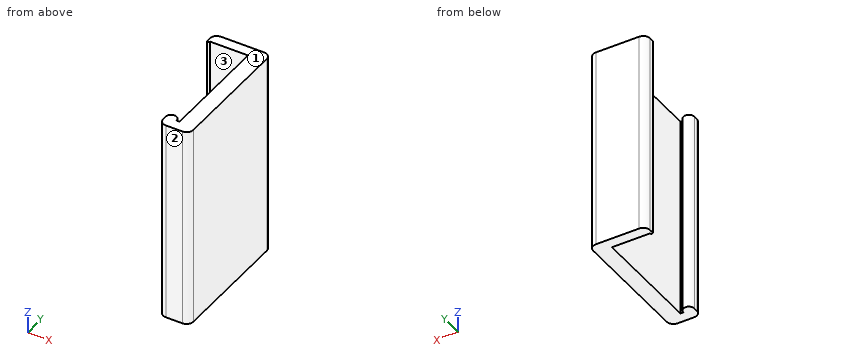
```python
from build123d import *

# Parameters (mm, degrees)
BOSS_EXTRUDE1_DEPTH      = 7.5
BOSS_EXTRUDE1_DEPTH_BACK = 7.5
FILLET1_R                = 0.5


with BuildPart() as part:
    # Sketch2 → Boss-Extrude1 (new, two sides: drawn at the far end of the back side and taken through both)
    with BuildSketch(Plane.XY.offset(-BOSS_EXTRUDE1_DEPTH_BACK)):
        Polygon((37.341321959, 6.45), (40.341321959, 6.45), (40.341321959, -1.8), (39.316321959, -1.8), (39.316321959, -2.6), (41.541321959, -2.6), (41.541321959, 7.25), (37.341321959, 7.25), align=None)
        with BuildLine():
            Line((37.541321959, 6.45), (37.341321959, 6.45))
            ThreePointArc((37.341321959, 6.45), (37.441321959, 6.35), (37.541321959, 6.45))
        make_face()
        with BuildLine():
            ThreePointArc((40.116321959, -1.8), (39.716321959, -1.4), (39.316321959, -1.8))
            Line((39.316321959, -1.8), (40.116321959, -1.8))
        make_face()
    extrude(amount=BOSS_EXTRUDE1_DEPTH + BOSS_EXTRUDE1_DEPTH_BACK)

    # Fillet1
    fillet1_edges = [part.edges().sort_by_distance(p)[0] for p in [
        (37.341321959, 7.25, 0),
        (41.541321959, 7.25, 0),
        (41.541321959, -2.6, 0),
        (39.316321959, -2.6, 0),
    ]]
    fillet(fillet1_edges, radius=FILLET1_R)


solid = part.part
```
Geometry check sheet. Reference: the model listing, model coordinates, mm. Face numbers are marked on the shaded views. Give positions to 0.01 mm unless a question says otherwise; leave off trailing zeros. Write each loop counter-clockwise with the first axis right and the second up, starting at its lowest first coordinate (ties: lowest second). Pieces come first, ordered by that corner, then holes. Notation, with made-up numbers: (2.25, 13) -> (17.25, 13) arc R26 cw to (17.25, 46) -> close; hole circle Ø8 at (37, 88.25). An arc over 180 degrees is marked (long way). Use one line per item in the form item = value.
Item 1: Sectioned sample at A-A on z = 6.5. Enter the section's corners in (x, y), plus the area to 3 significant figures.
Results list:
outline = (37.34, 6.45) arc R0.1 ccw to (37.54, 6.45) -> (40.34, 6.45) -> (40.34, -1.8) -> (40.12, -1.8) arc R0.4 ccw to (39.32, -1.8) -> (39.32, -2.1) arc R0.5 ccw to (39.82, -2.6) -> (41.04, -2.6) arc R0.5 ccw to (41.54, -2.1) -> (41.54, 6.75) arc R0.5 ccw to (41.04, 7.25) -> (37.84, 7.25) arc R0.5 ccw to (37.34, 6.75) -> close
area = 15.1 mm2
Item 2: Sectioned sample at B-B on x = 38.5. Enter the section's corners in (y, z), plus the area to 3 significant figures.
Results list:
outline = (6.45, -7.5) -> (7.25, -7.5) -> (7.25, 7.5) -> (6.45, 7.5) -> close
area = 12.0 mm2
Item 3: Scan lines: line 1 (Y direction, x = 39.75, z = -6.5); line 2 (X direction, y = 3.5, z = -3.5); line 3 (Y direction, x = 37.8, z = -6.25). Record each from-to range of solid material in increasing order.
Results list:
line_1 = -2.6 to -1.4, 6.45 to 7.25
line_2 = 40.34 to 41.54
line_3 = 6.45 to 7.25
Item 4: Sectioned sample at C-C on y = 1.5. Enter the section's corners in (x, z).
Results list:
outline = (40.34, -7.5) -> (41.54, -7.5) -> (41.54, 7.5) -> (40.34, 7.5) -> close
Item 5: Mould release check, pull along Y, two halves, no side actions. Record for the marked faces 1, 2 and 3: released by +Y, released by -Y, zero draft, split by the parting line, or undercut.
Results list:
face_1 = zero draft
face_2 = released by -Y
face_3 = undercut
Item 6: Depth check by flat-ended pin: pin 1 Ø1 at (x, y) = (40, 2.5) entering from +Z; pin 2 Ø1 at (x, y) = (38.5, 3) entering from +Z; pin 3 Ø3 at (y, z) = (3, 1.5) entering from -X. Enter the tip coordinate at first touch or a pass-through.
Results list:
pin_1 = 7.5
pin_2 = through
pin_3 = 40.34
